Geometry check sheet. Reference: drawing and pictorial views, mm from the part's lowest x, y, z. A direction names the side the tool comes from. Give positions to 0.01 mm unless a question says otherwise; leave off trailing zeros. Order: outer loops, then holes, each group sorted by start corner. A loop starts at its lowest first (then second) coordinate and runs counter-clockwise, first axis right, second up.
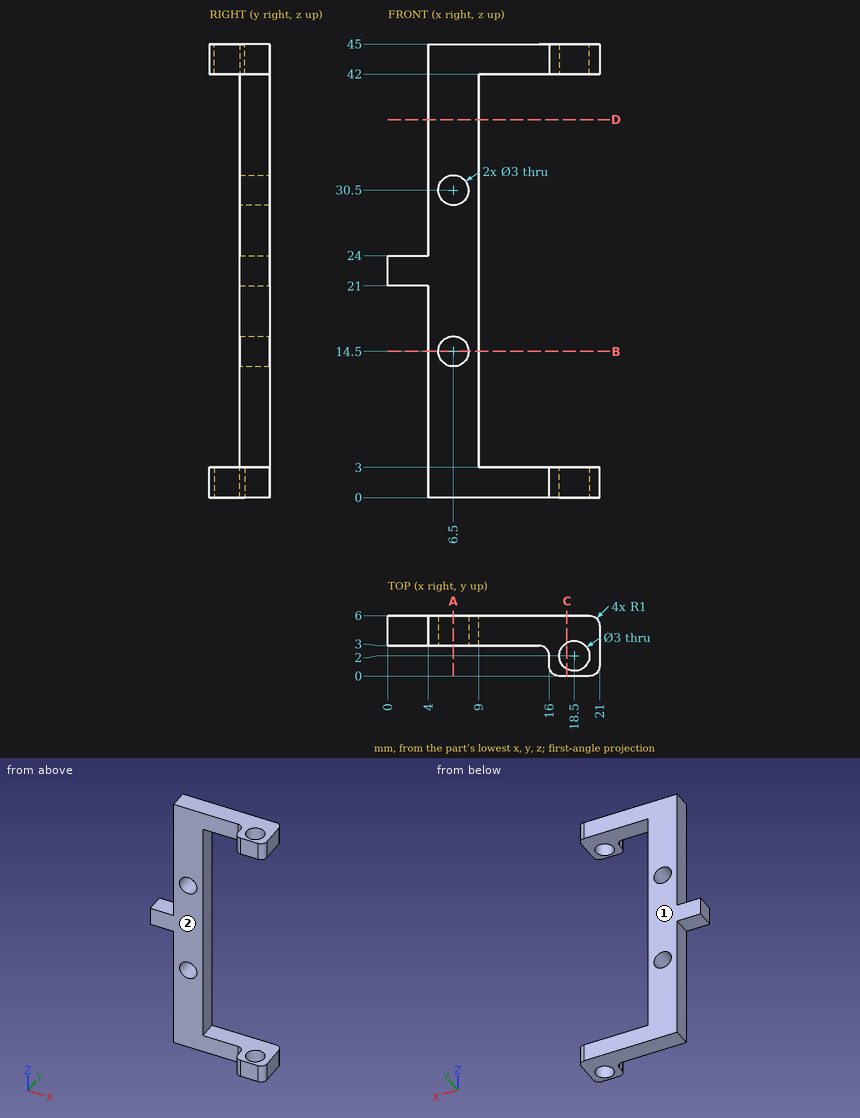
(1) Sectioned sample at A-A (x = 6.5). Enter the section's corners in (y, z), plus the area to 3 significant figures.
(2) Sectioned sample at D-D (z = 37.5). Enter the section's corners in (x, y).
(3) Tool access check on the marked faces 1 and 2. Record the directions out of +Z, -Z, +X, -X, +Y, -Y that give a thin tool (end or side, any length) a straight path to the whole face; none if there is none.
(4) Go/stop test with flat-tipped pins: P1, Ø1.5, axis at y = 5, z = 21.5, coming from the +X side; P2, Ø2, axis at x = 16, y = 2.5, coming from the -Z side; P3, Ø0.8, axis at y = 1.5, z = 43, coming from the -X side; P4, Ø3.5, axis at x = 6.5, z = 30.5, coming from the -Y side. Record where each tip stops, or that it passes through.
(5) Thickness scan on L1, parallel to Y at x = 18.5, z = 43; L2, parallel to X at y = 3.85, z = 30.5; L3, parallel to Z at x = 18.75, y = 4.9. Record the ranges inside material, lowest first.
(6) Sectioned sample at C-C (x = 17.75). Enter the section's corners in (y, z).
(7) Sectioned sample at B-B (z = 14.5). Enter the section's corners in (x, y).
Values follow:
1. outline: (3, 0) - (6, 0) - (6, 13) - (3, 13) - close; (3, 16) - (6, 16) - (6, 29) - (3, 29) - close; (3, 32) - (6, 32) - (6, 45) - (3, 45) - close
1. area: 117 mm2
2. outline: (4, 3) - (9, 3) - (9, 6) - (4, 6) - close
3. face 1: +Z, -Z, +X, -X, +Y
3. face 2: +Z, -Z, -X, -Y
4. P1: stops at x = 9
4. P2: stops at z = 0
4. P3: stops at x = 16
4. P4: stops at y = 3
5. L1: y = 0 to 0.5, 3.5 to 6
5. L2: x = 4 to 5, 8 to 9
5. L3: z = 0 to 3, 42 to 45
6. outline: (0, 0) - (0.7, 0) - (0.7, 3) - (0, 3) - close; (0, 42) - (0.7, 42) - (0.7, 45) - (0, 45) - close; (3.3, 0) - (6, 0) - (6, 3) - (3.3, 3) - close; (3.3, 42) - (6, 42) - (6, 45) - (3.3, 45) - close
7. outline: (4, 3) - (5, 3) - (5, 6) - (4, 6) - close; (8, 3) - (9, 3) - (9, 6) - (8, 6) - close
